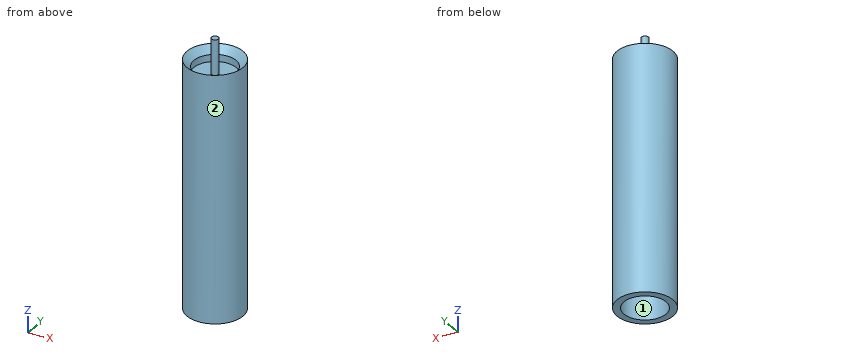
```python
from build123d import *

# Parameters (mm, degrees)
F0_R     = 4
F0_R_2   = 3
F1_DEPTH = 20
F2_DEPTH = 15
F3_DEPTH = 13
F4_SIZE  = 0.99999
F5_R     = 0.5
F6_DEPTH = 5


# Not quite as in the source:
# - a fillet or chamfer is up to 0.001 mm smaller than in the source, because OpenCascade refuses the exact size


with BuildPart() as f1:
    # F0 (on Top) → F1 (new body)
    with BuildSketch(Plane.XY):
        Circle(F0_R)
        Circle(F0_R_2, mode=Mode.SUBTRACT)
    extrude(amount=-F1_DEPTH)

    # F0 (on Top) → F2 (join)
    with BuildSketch(Plane.XY):
        Circle(F0_R)
        Circle(F0_R_2, mode=Mode.SUBTRACT)
    extrude(amount=F2_DEPTH)

    # F0 (on Top) → F3 (join)
    with BuildSketch(Plane.XY):
        Circle(F0_R_2)
    extrude(amount=F3_DEPTH)

    # F4 (size 1 in the source; OpenCascade refuses exactly that, so slightly less here)
    f4_edges = [f1.edges().sort_by_distance(p)[0] for p in [
        (-3, 0, 15),
    ]]
    chamfer(f4_edges, length=F4_SIZE)

    # F5 (on face) → F6 (join)
    with BuildSketch(Plane.XY.offset(13)):
        Circle(F5_R)
    extrude(amount=F6_DEPTH)


solid = f1.part
```
Model file for the job. Use its own axes, mm. Face numbers are marked on the shaded views. Coordinates: 2 decimals unless noted, no trailing zeros. Order: outer loops, then holes, each group sorted by start corner. A loop starts at its lowest first (then second) coordinate and runs counter-clockwise, first axis right, second up. Notation, with made-up numbers: (54.5, -29) -> (67.5, -29) arc R24 cw to (67.5, 10) -> close; hole circle Ø11 at (89, -6). An arc over 180 degrees is marked (long way). Return JSON: item names as keys, results as strings.
Item 1: Pin check, flat tips, straight feed: P1, Ø4, axis at y = -2.5, z = -15, coming from the +X side; P2, Ø3, axis at x = 1, y = 0, coming from the -Z side. Stop position of each tip, or through.
Model answer:
{"P1": "stops at x = 3.97", "P2": "stops at z = 0"}
Item 2: Slice it at D-D (z = 12). Write the cut outline in (x, y).
Model answer:
{"outline": "circle Ø8 at (0, 0)"}
Item 3: Wall check: line 1 along Y through (x, z) = (0, 13.55); line 2 along Z through (x, y) = (-1, 2.5); line 3 along Y through (x, z) = (0, -10.25). Give the ranges that are in metal, low to high. Write a range as from..to.
Model answer:
{"line 1": "y = -4..-3, -0.5..0.5, 3..4", "line 2": "z = 0..13", "line 3": "y = -4..-3, 3..4"}
Item 4: Slice it at C-C (z = -6). Write the cut outline in (x, y), then the cut area to 3 significant figures.
Model answer:
{"outline": "circle Ø8 at (0, 0); hole circle Ø6 at (0, 0)", "area": "22.0 mm²"}
Item 5: Mould opens along X. For the marked faces 1 and 2 say: pulls with the +X half, pulls with the -X half, needs draft (parallel to the pull), parting line crosses it, or undercut.
Model answer:
{"face 1": "undercut", "face 2": "parting line crosses it"}
